from build123d import *

# Parameters (mm, degrees)
F1_DEPTH = 5
F2_R     = 8.75
F3_DEPTH = 12.5
F5_DEPTH = 7.5
F7_DEPTH = 5
F8_R     = 10
F9_DEPTH = 25


with BuildPart() as f1:
    # F0 (on Top) → F1 (new body, symmetric)
    with BuildSketch(Plane.XY):
        with BuildLine():
            Line((20, -48.5), (20, 48.5))
            ThreePointArc((20, 48.5), (0, 68.5), (-20, 48.5))
            Line((-20, 48.5), (-20, -48.5))
            ThreePointArc((-20, -48.5), (0, -68.5), (20, -48.5))
        make_face()
    extrude(amount=F1_DEPTH, both=True)

    # F2 (on Top) → F3 (cut, symmetric)
    with BuildSketch(Plane.XY):
        with Locations((0, 20)):
            Circle(F2_R)
        with Locations((0, -20)):
            Circle(F2_R)
    extrude(amount=F3_DEPTH, both=True, mode=Mode.SUBTRACT)

    # F4 (on Top) → F5 (join, symmetric)
    with BuildSketch(Plane.XY):
        with BuildLine():
            Line((-15, 65), (-20, 65))
            Line((-20, 65), (-20, 20))
            Line((-20, 20), (-60, 20))
            ThreePointArc((-60, 20), (-80, 0), (-60, -20))
            Line((-60, -20), (-20, -20))
            Line((-20, -20), (-20, -55))
            Line((-20, -55), (-15, -55))
            Line((-15, -55), (-15, -21))
            ThreePointArc((-15, -21), (-10.313708499, -9.686291501), (1, -5))
            Line((1, -5), (20, -5))
            Line((20, -5), (20, 5))
            Line((20, 5), (1, 5))
            ThreePointArc((1, 5), (-10.313708499, 9.686291501), (-15, 21))
            Line((-15, 21), (-15, 65))
        make_face()
    extrude(amount=F5_DEPTH, both=True)

    # F6 (on Top) → F7 (cut, symmetric)
    with BuildSketch(Plane.XY):
        with BuildLine():
            Line((-35.5, 20), (-60, 20))
            ThreePointArc((-60, 20), (-80, 0), (-60, -20))
            Line((-60, -20), (-35.5, -20))
            Line((-35.5, -20), (-35.5, 20))
        make_face()
    extrude(amount=F7_DEPTH, both=True, mode=Mode.SUBTRACT)

    # F8 (on face) → F9 (cut)
    with BuildSketch(Plane.XY.offset(7.5)):
        with Locations((-60, 0)):
            Circle(F8_R)
    extrude(amount=-F9_DEPTH, mode=Mode.SUBTRACT)


solid = f1.part
The model under review builds one solid part; all positions refer to its coordinate system, in mm. A direction names the side the tool comes from. Round coordinates to 2 decimals unless told otherwise and drop trailing zeros. Write each loop counter-clockwise with the first axis right and the second up, starting at its lowest first coordinate (ties: lowest second). Pieces come first, ordered by that corner, then holes. Notation, with made-up numbers: M 88,80 L 128,80 A26 cw 128,99 Z; hole C -29.5,42.5 d9. An arc over 180 degrees is marked long. Answer as CSV lines item,"result". Start each with the question number.
Q1. Clearance check with flat-ended pins moving along their axes: P1, Ø11.5, axis at x = -4.5, y = -29, coming from the -Z side; P2, Ø6, axis at y = 48, z = -5, coming from the -X side; P3, Ø6, axis at x = -10.5, y = -15.5, coming from the +Z side. State where each tip first meets the part, or that it passes through.
Q2. Consider section D-D, the plane y = 33. Give the boundary of the cut face in (x, z), then the cut area to 3 significant figures.
Q3. Wall thickness on line 1 along Y through (x, z) = (0, 0.75); line 2 along Y through (x, z) = (-60, 6.6); line 3 along Z through (x, y) = (-49, -10): over which ranges is each line inside the solid? List them lowest first.
Q4. Tool access review of faces 5 (the face through (2, 37, 5)), 6 (the face through (-35, 20, 0)), 7 (the face through (-10.437, -9.811, -6.232)): name each direction out of +Z, -Z, +X, -X, +Y, -Y from which nothing blocks a thin tool from reaching the whole face with its end or side.
Q5. Consider section A-A, the plane y = 0. Give the boundary of the cut face in (x, z), then the cut area to 3 significant figures.
Q6. The part is to be moulded in two halves that separate along X. For faces 1 (the face through (-10.189, 9.563, 6.268)), 2 (the face through (-70, 0, 6)), 3 (the face through (2, 37, -5)), 4 (the face through (-1.139, 28.676, 0.07)), say which applies: +X half, -X half, draft (parallel to the pull), parting line (faces both ways), or undercut.
Q7. Consider section B-B, the plane x = -64. Give the boundary of the cut face in (y, z), then the cut area to 3 significant figures.
Q8. Consider section C-C, the plane x = -46. Give the boundary of the cut face in (y, z), then the cut area to 3 significant figures.
Result set:
1,P1,"stops at z = -5"
1,P2,"stops at x = -20"
1,P3,"stops at z = 5"
2,outline,"M -20,-7.5 L -15,-7.5 L -15,-5 L 20,-5 L 20,5 L -15,5 L -15,7.5 L -20,7.5 Z"
2,area,"425 mm²"
3,line 1,"y = -68.5 to -28.75, -11.25 to 11.25, 28.75 to 68.5"
3,line 2,"y = -20 to -10, 10 to 20"
3,line 3,"z = -7.5 to -5, 5 to 7.5"
4,face 5,"+Z, +X, +Y"
4,face 6,"+Z, -Z, -X, +Y"
4,face 7,"-Z, +X, -Y"
5,outline,"M -80,-7.5 L -70,-7.5 L -70,-5 L -80,-5 Z; M -80,5 L -70,5 L -70,7.5 L -80,7.5 Z; M -50,-7.5 L 20,-7.5 L 20,7.5 L -50,7.5 L -50,5 L -35.5,5 L -35.5,-5 L -50,-5 Z"
5,area,"955 mm²"
6,face 1,"+X half"
6,face 2,"undercut"
6,face 3,"draft"
6,face 4,"undercut"
7,outline,"M -19.6,-7.5 L -9.17,-7.5 L -9.17,-5 L -19.6,-5 Z; M -19.6,5 L -9.17,5 L -9.17,7.5 L -19.6,7.5 Z; M 9.17,-7.5 L 19.6,-7.5 L 19.6,-5 L 9.17,-5 Z; M 9.17,5 L 19.6,5 L 19.6,7.5 L 9.17,7.5 Z"
7,area,"104 mm²"
8,outline,"M -20,-7.5 L 20,-7.5 L 20,-5 L -20,-5 Z; M -20,5 L 20,5 L 20,7.5 L -20,7.5 Z"
8,area,"200 mm²"
